Input: dimensioned drawing with shaded views. Units: mm. Origin: part minimum x, y, z. A direction names the side the tool comes from. Give positions to 0.01 mm unless a question says otherwise; leave off trailing zeros. Write each loop counter-clockwise with the first axis right and the second up, starting at its lowest first coordinate (ties: lowest second). Pieces come first, ordered by that corner, then holes. Notation, with made-up numbers: (4, 61.5) -> (56, 61.5) arc R27 ccw to (56, 96.5) -> close; hole circle Ø4 at (12.25, -21). An arc over 180 degrees is marked (long way). Answer as a JSON object with one key per item and string values. Group by question number.
(1) Section query B-B on z = 2. Output: boundary loops of the cut face in (x, y).
(2) Section query D-D on x = 50. Output: boundary loops of the cut face in (y, z).
(3) Draft query along X for the marked faces 1, 2 and 3. Return one class per face: +X half, -X half, draft (parallel to the pull), parting line (faces both ways), or undercut.
(4) Contact query for flat-ended pins moving along their axis: pin 1 Ø1.6 at (x, z) = (11.5, 7.5) entering from -Y; pin 2 Ø1.5 at (x, z) = (15.5, 2.5) entering from -Y; pin 3 Ø1.2 at (y, z) = (7, 4.5) entering from +X. Output: stop coordinate, or through.
(5) Section query C-C on x = 8. Output: boundary loops of the cut face in (y, z).
(6) Section query A-A on y = 16. Output: boundary loops of the cut face in (x, z).
(7) Material intervals for probe 1 along Y at (x, z) = (24, 8); probe 2 along Y at (x, z) = (49, 2); probe 3 along X at (y, z) = (3.5, 0.5), sorted ascending.
(8) Set-up query: the marked faces 4 and 5. Return all of +Z, -Z, +X, -X, +Y, -Y with unobstructed straight access to the full face (end or side cutting, diameter ignored); none if empty.
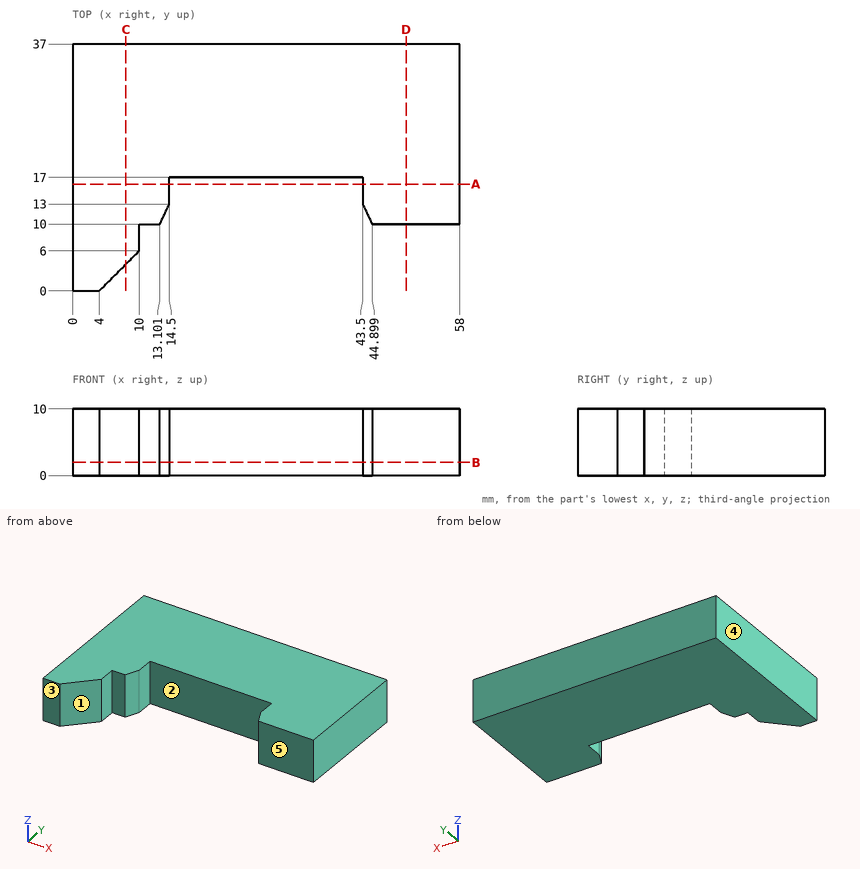
Answer list:
{
 "1": {"outline": "(0, 0) -> (4, 0) -> (10, 6) -> (10, 10) -> (13.1, 10) -> (14.5, 13) -> (14.5, 17) -> (43.5, 17) -> (43.5, 13) -> (44.9, 10) -> (58, 10) -> (58, 37) -> (0, 37) -> close"},
 "2": {"outline": "(10, 0) -> (37, 0) -> (37, 10) -> (10, 10) -> close"},
 "3": {"face 1": "+X half", "face 2": "undercut", "face 3": "draft"},
 "4": {"pin 1": "y = 10", "pin 2": "y = 17", "pin 3": "x = 10"},
 "5": {"outline": "(4, 0) -> (37, 0) -> (37, 10) -> (4, 10) -> close"},
 "6": {"outline": "(0, 0) -> (14.5, 0) -> (14.5, 10) -> (0, 10) -> close; (43.5, 0) -> (58, 0) -> (58, 10) -> (43.5, 10) -> close"},
 "7": {"probe 1": "17 to 37", "probe 2": "10 to 37", "probe 3": "0 to 7.5"},
 "8": {"face 4": "+Z, -Z, -X, +Y, -Y", "face 5": "+Z, -Z, +X, -Y"}
}
